Autodesk Inventor part; units mm, degrees
ref_plane "YZ Plane" through (0, 0, 0) normal (1, 0, 0) x (0, 1, 0)
ref_plane "XZ Plane" through (0, 0, 0) normal (0, 1, 0) x (-1, 0, 0)
ref_plane "XY Plane" through (0, 0, 0) normal (0, 0, 1) x (1, 0, 0)
sketch "Sketch1" plane through (0, 0, 0) normal (0, 1, 0) x (-1, 0, 0)
  line L0 (0, 0) -> (-149.225, 0)
  line L1 (-149.225, 0) -> (-149.225, -149.225)
  line L2 (-149.225, -149.225) -> (0, -149.225)
  line L3 (0, -149.225) -> (0, 0)
  circle A0 centre (-74.6125, -74.6125) radius 14.351
  dimension "d0" = 149.225
  dimension "d1" = 149.225
  dimension "d2" = 28.702
extrude "Extrusion1" add sketch "Sketch1" along normal blind 2.2098
sketch "Sketch5" plane through (0, 2.2098, 0) normal (0, 1, 0) x (1, 0, 0)
  circle A0 centre (74.6125, 74.6125) radius 14.351
  line L0 (0, 0) -> (149.225, 0)
  line L1 (149.225, 0) -> (149.225, 149.225)
  line L2 (149.225, 149.225) -> (0, 149.225)
  line L3 (0, 149.225) -> (0, 0)
  line L4 (0, 0) -> (114.3, 0)
  line L5 (114.3, 0) -> (114.3, 257.2258)
  line L6 (114.3, 257.2258) -> (0, 257.2258)
  line L7 (0, 257.2258) -> (0, 0)
  dimension "d21" = 114.3
  dimension "d22" = 257.2258
extrude "Extrusion6" add sketch "Sketch5" against normal blind 2.2098 contours L3 L2 L5 L0 | L7 L6 L5 L2
sketch "Sketch6" plane through (0, 2.2098, 0) normal (0, 1, 0) x (1, 0, 0)
  line L0 (114.3, 149.225) -> (149.225, 149.225)
  line L1 (149.225, 149.225) -> (149.225, 0)
  line L2 (149.225, 0) -> (114.3, 0)
  line L3 (114.3, 0) -> (114.3, 149.225)
  point P0 (0, 0)
extrude "Extrusion7" cut sketch "Sketch6" against normal blind 2.2098
sketch "Sketch7" plane through (0, 2.2098, 0) normal (0, 1, 0) x (1, 0, 0)
  circle A0 centre (74.6125, 74.6125) radius 14.351
  circle A1 centre (74.6125, 74.6125) radius 14.351
  point P0 (0, 0)
extrude "Extrusion8" add sketch "Sketch7" against normal blind 2.2098
sketch "Sketch8" plane through (0, 2.2098, 0) normal (0, 1, 0) x (1, 0, 0)
  line L0 (0, 0) -> (114.3, 0)
  line L1 (16.637, 0) -> (97.663, 0)
  line L2 (16.637, 30.422) -> (16.637, 0)
  line L3 (16.637, 40.513) -> (57.15, 40.513)
  line L4 (57.15, 40.513) -> (57.15, 0)
  line L5 (57.15, 0) -> (16.637, 0)
  line L6 (16.637, 0) -> (16.637, 40.513)
  circle A0 centre (57.15, 40.513) radius 15.494
  dimension "d31" = 30.988
extrude "Extrusion9" cut sketch "Sketch8" against normal blind 2.2098 contours A0 L3 L4 | L4 L3 A0
sketch "Sketch9" plane through (0, 2.2098, 0) normal (0, 1, 0) x (1, 0, 0)
  circle A0 centre (57.15, 40.513) radius 15.494
  line L0 (114.3, 0) -> (114.3, 257.2258)
  line L1 (114.3, 257.2258) -> (0, 257.2258)
  line L2 (0, 257.2258) -> (0, 0)
  line L3 (0, 0) -> (114.3, 0)
  line L4 (0, 0) -> (114.3, 0)
  line L5 (114.3, 0) -> (114.3, -25.4)
  line L6 (114.3, -25.4) -> (0, -25.4)
  line L7 (0, -25.4) -> (0, 0)
  line L8 (114.3, 257.2258) -> (114.3, 0)
  line L9 (0, 257.2258) -> (114.3, 257.2258)
  line L10 (114.3, 257.2258) -> (114.3, 231.8258)
  line L11 (114.3, 231.8258) -> (0, 231.8258)
  line L12 (0, 231.8258) -> (0, 257.2258)
  dimension "d34" = 25.4
  dimension "d35" = 25.4
extrude "Extrusion10" cut sketch "Sketch9" against normal blind 2.2098 contours L11 L2 L1 L0
extrude "Extrusion11" add sketch "Sketch9" against normal blind 2.2098 contours L5 L6 L7 L3
sketch "Sketch10" plane through (0, 2.2098, 0) normal (0, 1, 0) x (1, 0, 0)
  line L0 (0, -25.4) -> (25.4, -25.4)
  line L1 (25.4, -25.4) -> (25.4, 86.8868)
  line L2 (25.4, 86.8868) -> (0, 86.8868)
  line L3 (0, 86.8868) -> (0, -25.4)
  line L4 (114.3, -25.4) -> (114.3, 231.8258)
  line L5 (0, -25.4) -> (114.3, -25.4)
  line L6 (114.3, -25.4) -> (114.3, 0)
  line L7 (114.3, 0) -> (0, 0)
  line L8 (0, 0) -> (0, -25.4)
  line L9 (114.3, 231.8258) -> (0, 231.8258)
  line L10 (0, 231.8258) -> (0, -25.4)
  line L11 (0, -25.4) -> (114.3, -25.4)
  line L12 (114.3, -25.4) -> (114.3, 231.8258)
  circle A0 centre (57.15, 40.513) radius 15.494
  circle A1 centre (57.15, 40.513) radius 15.494
  dimension "d40" = 25.4
extrude "Extrusion12" add sketch "Sketch10" against normal blind 2.2098 contours A0
sketch "Sketch11" plane through (0, 2.2098, 0) normal (0, 1, 0) x (1, 0, 0)
  line L0 (25.3965, 0) -> (68.5765, 0)
  line L1 (68.5765, 0) -> (68.5765, 43.18)
  line L2 (68.5765, 43.18) -> (25.3965, 43.18)
  line L3 (25.3965, 43.18) -> (25.3965, 0)
  circle A0 centre (68.5765, 43.18) radius 15.494
  point P0 (0, 0)
  dimension "d43" = 43.18
  dimension "d44" = 43.18
  dimension "d45" = 30.988
extrude "Extrusion13" cut sketch "Sketch11" against normal blind 2.2098 contours A0 L2 L1 | L1 L2 A0
sketch "Sketch12" plane through (0, 2.2098, 0) normal (0, 1, 0) x (1, 0, 0)
  circle A0 centre (68.5765, 43.18) radius 15.494
  line L0 (114.3, 231.8258) -> (0, 231.8258)
  line L1 (0, 231.8258) -> (0, -25.4)
  line L2 (0, -25.4) -> (114.3, -25.4)
  line L3 (114.3, -25.4) -> (114.3, 231.8258)
  line L4 (0, 231.8258) -> (114.3, 231.8258)
  line L5 (114.3, 231.8258) -> (114.3, 257.2258)
  line L6 (114.3, 257.2258) -> (0, 257.2258)
  line L7 (0, 257.2258) -> (0, 231.8258)
  point P0 (0, 0)
  dimension "d48" = 25.4
extrude "Extrusion14" add sketch "Sketch12" against normal blind 2.2098 contours L0 L7 L6 L5
properties part number "bearing plate"
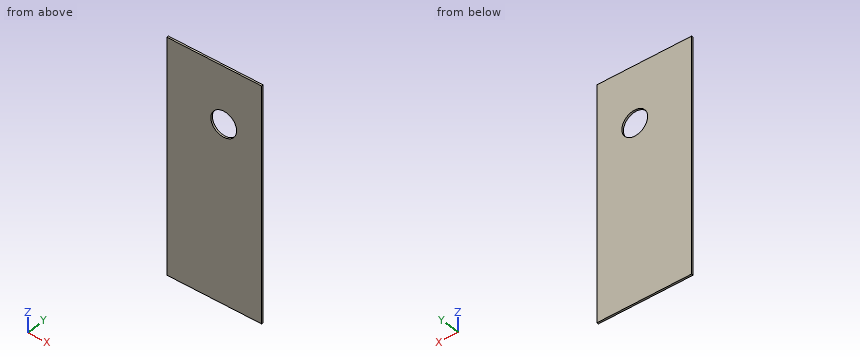
The listing builds one solid part. Answer for the finished solid, in the listing's coordinates (mm). Coordinates: 2 decimals unless noted, no trailing zeros. Write each loop counter-clockwise with the first axis right and the second up, starting at its lowest first coordinate (ties: lowest second). Pieces come first, ordered by that corner, then holes. Notation, with made-up numbers: (68.25, 32.5) -> (103.25, 32.5) arc R22 cw to (103.25, 62.5) -> close; hole circle Ø4 at (0.5, -16.5). An arc over 180 degrees is marked (long way). Write each question's results on one line, items separated by ' | '. Start each with the question number.
1) A cutting plane is placed at A-A (z = -43.18). Determine the outline of the cut face in (x, y).
2) A flat-ended cylindrical pin translates along its axis: pin 1 Ø18.5 at (x, z) = (68.58, -43.18) entering from +Y. Find the tip coordinate at first contact, or state that the pin passes through.
3) Straight lines are drawn through the part: probe 1 along X at (y, z) = (0.7, -43.18); probe 2 along X at (y, z) = (0.25, -29); probe 3 along Z at (x, y) = (57, 0.5). For each, find the intervals that lie inside material, in ascending order.
4) A cutting plane is placed at B-B (y = 0.65). Determine the outline of the cut face in (x, z), then the cut area to 4 significant figures.
5) A cutting plane is placed at C-C (x = 74). Determine the outline of the cut face in (y, z).
Values follow:
1) outline: (0, 0) -> (53.08, 0) -> (53.08, 2.21) -> (0, 2.21) -> close; (84.07, 0) -> (114.3, 0) -> (114.3, 2.21) -> (84.07, 2.21) -> close
2) pin 1: through
3) probe 1: 0 to 53.08, 84.07 to 114.3 | probe 2: 0 to 62.33, 74.82 to 114.3 | probe 3: -257.23 to -53.48, -32.88 to 25.4
4) outline: (0, -257.23) -> (114.3, -257.23) -> (114.3, 25.4) -> (0, 25.4) -> close; hole circle Ø30.99 at (68.58, -43.18) | area: 31,550 mm²
5) outline: (0, -257.23) -> (2.21, -257.23) -> (2.21, -57.69) -> (0, -57.69) -> close; (0, -28.67) -> (2.21, -28.67) -> (2.21, 25.4) -> (0, 25.4) -> close
